Autodesk Inventor part; units mm, degrees
ref_plane "YZ Plane" through (0, 0, 0) normal (1, 0, 0) x (0, 1, 0)
ref_plane "XZ Plane" through (0, 0, 0) normal (0, 1, 0) x (-1, 0, 0)
ref_plane "XY Plane" through (0, 0, 0) normal (0, 0, 1) x (1, 0, 0)
sketch "スケッチ1" plane through (0, 0, 0) normal (0, 0, 1) x (1, 0, 0)
  circle A0 centre (68, 27) radius 4.05
  circle A1 centre (31, -5) radius 4.05
  circle A2 centre (48, -5) radius 4.05
  circle A3 centre (68, 27) radius 6.5 construction
  circle A4 centre (31, -5) radius 6.5 construction
  circle A5 centre (48, -5) radius 6.5 construction
  line L0 (31, -11.5) -> (48, -11.5)
  line L1 (73.512, 23.555) -> (53.512, -8.445)
  arc A6 (48, -11.5) -> (53.512, -8.445) centre (48, -5) ccw
  circle A7 centre (39, 13.5) radius 1.35
  line L2 (39, 13.5) -> (39, 40.5) construction
  line L3 (39, 40.5) -> (12, 40.5) construction
  line L4 (12, 40.5) -> (12, 13.5) construction
  line L5 (12, 13.5) -> (39, 13.5) construction
  circle A8 centre (12, 13.5) radius 1.35
  circle A9 centre (12, 40.5) radius 1.35
  circle A10 centre (39, 40.5) radius 1.35
  circle A11 centre (11, 27) radius 8.5 construction
  circle A12 centre (11, 27) radius 10.5 construction
  arc A13 (0, 15.381) -> (0, 38.619) centre (11, 27) ccw construction
  line L6 (0, 15.381) -> (0, 38.619) construction
  line L7 (11, 11) -> (11, 43) construction
  line L8 (11, 43) -> (51.5, 43) construction
  line L9 (51.5, 43) -> (51.5, 11) construction
  line L10 (51.5, 11) -> (11, 11) construction
  circle A14 centre (39, 13.5) radius 2.5 construction
  circle A15 centre (39, 40.5) radius 2.5 construction
  circle A16 centre (12, 40.5) radius 2.5 construction
  circle A17 centre (12, 13.5) radius 2.5 construction
  line L11 (10.0057, 11.9924) -> (25.8149, -8.9198)
  line L12 (69.9848, 33.1896) -> (39.7634, 42.8806)
  arc A18 (25.8149, -8.9198) -> (31, -11.5) centre (31, -5) ccw
  arc A19 (12, 16) -> (10.0057, 11.9924) centre (12, 13.5) ccw
  arc A20 (12, 16) -> (12, 38) centre (11, 27) ccw
  line L13 (12, 43) -> (39, 43)
  arc A21 (39.7634, 42.8806) -> (39, 43) centre (39, 40.5) ccw
  arc A22 (73.512, 23.555) -> (69.9848, 33.1896) centre (68, 27) ccw
  arc A23 (12, 43) -> (12, 38) centre (12, 40.5) ccw
  point P0 (0, 0)
  point P1 (62.8293, 30.9388)
  point P2 (24.5, -5)
  point P3 (1.5716, 22.3787)
  point P4 (39, 11)
  dimension "d60" = 21
  dimension "d17" = 8.1
  dimension "d21" = 5
  dimension "d24" = 17
  dimension "d26" = 20
  dimension "d27" = 13
  dimension "d55" = 2.7
  dimension "d56" = 27
  dimension "d57" = 27
  dimension "d58" = 17
  dimension "d59" = 1
  dimension "d61" = 32
  dimension "d62" = 13.5
  dimension "d63" = 12
  dimension "d64" = 51.5
  dimension "d65" = 5
  dimension "d66" = 57
  dimension "d67" = 32
  dimension "d68" = 32
  dimension "d69" = 20
extrude "押し出し1" add sketch "スケッチ1" along normal blind 2
sketch "スケッチ5" plane through (0, 0, 2) normal (0, 0, 1) x (1, 0, 0)
  circle A0 centre (12, 40.5) radius 1.35
  circle A1 centre (39, 40.5) radius 1.35
  circle A2 centre (39, 13.5) radius 1.35
  circle A3 centre (12, 13.5) radius 1.35
  circle A4 centre (31, -5) radius 4.05
  circle A5 centre (48, -5) radius 4.05
  circle A6 centre (68, 27) radius 4.05
  line L0 (39, 43) -> (12, 43)
  circle A7 centre (12, 40.5) radius 2.5 construction
  circle A8 centre (39, 40.5) radius 2.5 construction
  circle A9 centre (39, 13.5) radius 2.5 construction
  circle A10 centre (12, 13.5) radius 2.5 construction
  circle A11 centre (31, -5) radius 6.5 construction
  circle A12 centre (48, -5) radius 6.5 construction
  circle A13 centre (68, 27) radius 6.5 construction
  arc A14 (73.512, 23.555) -> (69.9848, 33.1896) centre (68, 27) ccw
  line L1 (14.5, 40.5) -> (36.5, 40.5)
  line L2 (36.5, 40.5) -> (36.5, 13.5)
  line L3 (14.5, 13.5) -> (36.5, 13.5)
  arc A15 (12, 16) -> (12, 38) centre (11, 27) ccw
  arc A16 (14.5, 13.5) -> (14.5, 40.5) centre (11, 27) ccw
  line L4 (40.4464, 38.4609) -> (42.5, 37.8024)
  line L5 (69.9848, 33.1896) -> (39.7634, 42.8806)
  line L6 (68, 27) -> (11, 27) construction
  line L7 (63.0499, 22.7873) -> (42.5, 16.1976)
  line L8 (42.5, 37.8024) -> (42.5, 28.25)
  line L9 (39.7634, 11.1194) -> (42.5098, 12.0001)
  arc A17 (63.0499, 31.2127) -> (61.6213, 28.25) centre (68, 27) ccw
  line L10 (39, 13.5) -> (48, -5) construction
  line L11 (39, 13.5) -> (31, -5) construction
  line L12 (41.2481, 14.5937) -> (42.5098, 12.0001)
  line L13 (36.7519, 12.4063) -> (39.1337, 7.5105)
  line L14 (41.2946, 12.5077) -> (39.1337, 7.5105)
  line L15 (65.92, 20.8418) -> (64.8766, 19.1724)
  line L16 (53.512, -8.445) -> (73.512, 23.555)
  arc A18 (52.624, -0.4318) -> (47.6233, 1.4891) centre (48, -5) ccw
  line L17 (10.0057, 11.9924) -> (25.8149, -8.9198)
  line L18 (37.5, -5) -> (41.5, -5)
  arc A19 (43.1271, -0.6983) -> (41.5, -5) centre (48, -5) ccw
  arc A20 (37.5, -5) -> (35.6761, -0.4851) centre (31, -5) ccw
  arc A21 (31.0868, 1.4994) -> (25.9894, -0.8594) centre (31, -5) ccw
  line L19 (31, -5) -> (48, -5) construction
  line L20 (39.1337, 7.5105) -> (43.1271, -0.6983)
  line L21 (39.1337, 7.5105) -> (35.6761, -0.4851)
  line L22 (42.5098, 12.0001) -> (64.8766, 19.1724)
  line L23 (42.5098, 12.0001) -> (47.6233, 1.4891)
  line L24 (42.5, 16.1976) -> (40.4464, 15.5391)
  line L25 (42.5, 37.8024) -> (63.0499, 31.2127)
  line L26 (64.8766, 19.1724) -> (69.9848, 20.8104)
  line L27 (64.8766, 19.1724) -> (52.624, -0.4318)
  line L28 (36.0599, 11) -> (35.1952, 11)
  line L29 (36.7054, 14.4923) -> (35.1952, 11)
  line L30 (25.9894, -0.8594) -> (17.0239, 11)
  line L31 (17.0239, 11) -> (13.9943, 15.0076)
  line L32 (17.0239, 11) -> (14.4985, 11)
  line L33 (35.1952, 11) -> (17.0239, 11)
  line L34 (35.1952, 11) -> (31.0868, 1.4994)
  line L35 (61.6213, 28.25) -> (42.5, 28.25)
  line L36 (61.6213, 25.75) -> (42.5, 25.75)
  arc A22 (61.6213, 28.25) -> (61.6213, 25.75) centre (68, 27) ccw construction
  arc A23 (61.6213, 25.75) -> (63.0499, 22.7873) centre (68, 27) ccw
  line L37 (42.5, 28.25) -> (42.5, 25.75) construction
  line L38 (42.5, 25.75) -> (42.5, 16.1976)
  point P0 (0, 0)
  dimension "d71" = 4
  dimension "d73" = 5
  dimension "d75" = 5
  dimension "d81" = 6
  dimension "d82" = 2.5
  dimension "d83" = 5
  dimension "d84" = 5
  dimension "d85" = 2.5
extrude "押し出し3" cut sketch "スケッチ5" against normal through all contours L1 L2 L29 L3 L31 A16 | L31 L3 A16 | L2 L3 L29 | L33 L34 A21 L30 | L7 L38 L36 A23 | L25 A17 L35 L8 | L22 L27 A18 L23 | L20 A19 L18 A20 L21
fillet "フィレット2" radius 3 25 edges at (36.5, 13.5, 1) (39.1337, 7.5105, 1) (42.5098, 12.0001, 1) (35.6761, -0.4851, 1) (37.5, -5, 1) (43.1271, -0.6983, 1) (41.5, -5, 1) (47.6233, 1.4891, 1) (52.624, -0.4318, 1) (64.8766, 19.1724, 1) (63.0499, 22.7873, 1) (63.0499, 31.2127, 1) (42.5, 37.8024, 1) (36.5, 40.5, 1) (31.0868, 1.4994, 1) (25.9894, -0.8594, 1) (42.5, 16.1976, 1) (14.5, 13.5, 1) (14.5, 40.5, 1) (35.1952, 11, 1) (17.0239, 11, 1) (42.5, 25.75, 1) (42.5, 28.25, 1) (61.6213, 28.25, 1) (61.6213, 25.75, 1)
equation "\"d62\" = 0.5 * d56"
equation "\"d45\" = d44"
properties part number "膝_メインフレーム" material "アルミニウム 2014-T4"
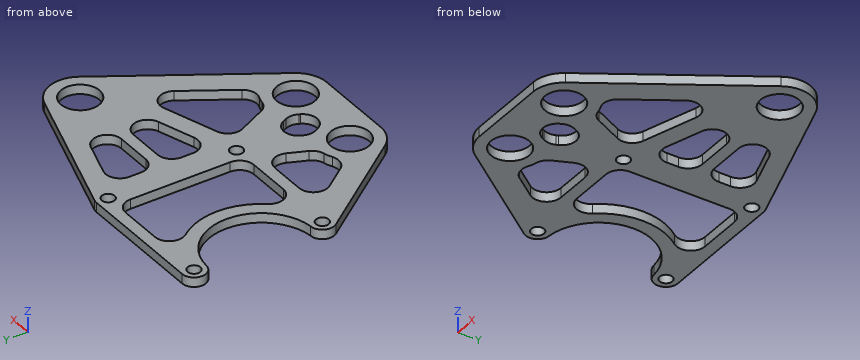
Read the model definition and answer for the solid it produces. Units are mm, in the model's axes. Coordinates: 2 decimals unless noted, no trailing zeros. Order: outer loops, then holes, each group sorted by start corner. A loop starts at its lowest first (then second) coordinate and runs counter-clockwise, first axis right, second up. Notation, with made-up numbers: M 8.25,16 L 19.25,16 A11 ccw 19.25,20 Z; hole C -17.5,3 d10. An arc over 180 degrees is marked long. Put each result on its own line as item: value. Start each with the question number.
Item 1: Given pin 1 Ø6.5 at (x, y) = (31, -5) entering from +Z; pin 2 Ø1 at (x, z) = (19, 0.5) entering from -Y; pin 3 Ø1 at (x, z) = (27.5, 1) entering from -Y, each flat-ended and moving along its own axis, determine where each tip first touches the part or whether it passes through.
Item 2: Section A-A, the plane x = 68 is taken. Determine the outline of the cut face in (y, z), plus the area to 3 significant figures.
Item 3: Consider probe 1 along Y at (x, z) = (48, 0.85); probe 2 along X at (y, z) = (-6.5, 1.75); probe 3 along Y at (x, z) = (26, 0.8). Determine where each line is inside the solid, lowest interval first. Write a range as [from, to].
Item 4: Section B-B, the plane z = 1.45 is taken. Count the separate pieces of the cut face and the enclosed holes in it, plus the area to 3 significant figures.
Computed:
1. pin 1: passes through
1. pin 2: stops at y = -0.57
1. pin 3: stops at y = -10.77
2. outline: M 14.74,0 L 22.95,0 L 22.95,2 L 14.74,2 Z; M 31.05,0 L 33.83,0 L 33.83,2 L 31.05,2 Z
2. area: 22.0 mm2
3. probe 1: y = [-11.5, -9.05], [-0.95, 1.81], [13.76, 17.96], [25.75, 28.25], [36.04, 40.24]
3. probe 2: x = [23.99, 27.24], [34.76, 44.24], [51.76, 54.73]
3. probe 3: y = [-9.15, 0.44], [11, 13.5], [40.5, 43]
4. separate pieces: 1
4. enclosed holes: 13
4. area: 1,430 mm2
